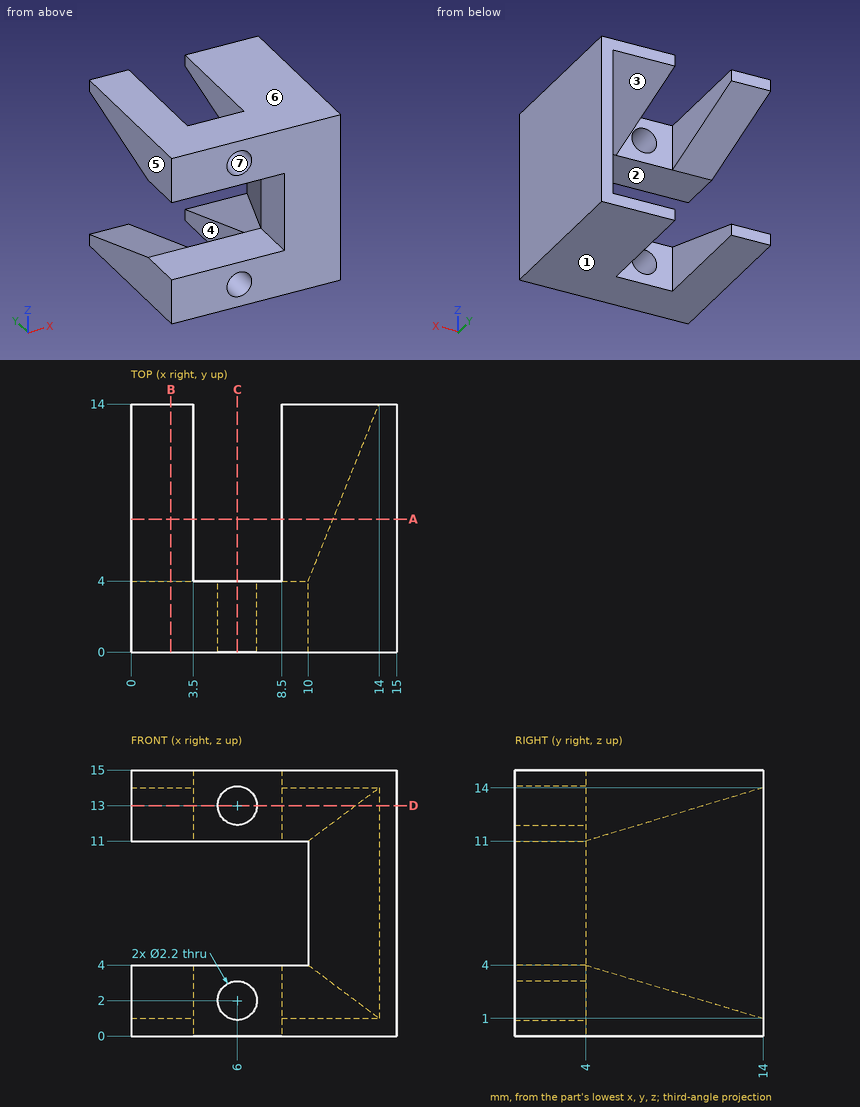
Print and shaded views of the part. All mm, measured from the part's lowest x, y and z. A direction names the side the tool comes from. Coordinates: 2 decimals unless noted, no trailing zeros. Order: outer loops, then holes, each group sorted by start corner. A loop starts at its lowest first (then second) coordinate and runs counter-clockwise, first axis right, second up. Notation, with made-up numbers: M -28,-12.5 L -15,-12.5 A25 ccw -15,5.5 Z; hole C -6.75,85.5 d9. An arc over 180 degrees is marked long. Write each question's results on one line, items separated by ' | '. Start each with the question number.
Q1. Cut at A-A (y = 7.5). List the corners of the cut face in (x, z), then the cut area to 3 significant figures.
Q2. Cut at D-D (z = 13). List the corners of the cut face in (x, y), then the cut area to 3 significant figures.
Q3. Drill centre lines: probe 1 along Z at (x, y) = (6.5, 3.5); probe 2 along Z at (x, y) = (9.75, 1); probe 3 along X at (y, z) = (1.9, 13). Where is each one in solid material? Low to high. Write a range as from..to.
Q4. Pull direction Z, two halves, no side cores. Call the marked faces 5, 6 and 7: +Z half, -Z half, draft (parallel to the pull), parting line (faces both ways), or undercut.
Q5. Which spindle directions (+Z, -Z, +X, -X, +Y, -Y) get a long thin tool onto all of the face, cutting with end or side? Do the marked faces 1, 2, 3 and 4. Say none if no direction does.
Q6. Cut at C-C (x = 6). List the corners of the cut face in (y, z).
Q7. Cut at B-B (x = 2.25). List the corners of the cut face in (y, z), then the cut area to 3 significant figures.
Q8. Flat gauge pins, fed straight in: P1, Ø8, axis at x = 12.5, z = 2.5, coming from the -Y side; P2, Ø3.5, axis at x = 6, z = 13, coming from the +Y side; P3, Ø2, axis at y = 2, z = 8, coming from the -X side. Where does each tip first touch, or does it go through?
Found:
1) outline: M 0,0 L 3.5,0 L 3.5,2.95 L 0,2.95 Z; M 0,12.05 L 3.5,12.05 L 3.5,15 L 0,15 Z; M 8.5,0 L 15,0 L 15,15 L 8.5,15 L 8.5,12.05 L 11.4,12.05 L 11.4,2.95 L 8.5,2.95 Z | area: 91.8 mm²
2) outline: M 0,0 L 4.9,0 L 4.9,4 L 3.5,4 L 3.5,10.67 L 0,10.67 Z; M 7.1,0 L 15,0 L 15,14 L 14,14 L 12.67,10.67 L 8.5,10.67 L 8.5,4 L 7.1,4 Z | area: 123 mm²
3) probe 1: 0..1.02, 2.98..4, 11..12.02, 13.98..15 | probe 2: 0..4, 11..15 | probe 3: 0..4.9, 7.1..15
4) face 5: draft | face 6: +Z half | face 7: undercut
5) face 1: -Z, +X, -X, +Y, -Y | face 2: -X, +Y, -Y | face 3: -X, +Y | face 4: +Z, -Z, +Y
6) outline: M 0,0 L 4,0 L 4,0.9 L 0,0.9 Z; M 0,3.1 L 4,3.1 L 4,4 L 0,4 Z; M 0,11 L 4,11 L 4,11.9 L 0,11.9 Z; M 0,14.1 L 4,14.1 L 4,15 L 0,15 Z
7) outline: M 0,0 L 14,0 L 14,1 L 4,4 L 0,4 Z; M 0,11 L 4,11 L 14,14 L 14,15 L 0,15 Z | area: 82.0 mm²
8) P1: y = 0 | P2: y = 4 | P3: x = 10
